Input: part model. Units: mm. Frame: model coordinates. Coordinates: 2 decimals unless noted, no trailing zeros. Write each loop counter-clockwise with the first axis right and the second up, starting at its lowest first coordinate (ties: lowest second). Pieces come first, ordered by that corner, then holes.
1) Draft query along X for faces 1 (the flat face through (-6, 0, -3)), 2 (the cylindrical face through (-5.49, 0.2, -7.62)), 3 (the cylindrical face through (-1.59, 0.2, -3.16)). Return one class per face: pulls with the +X half, pulls with the -X half, needs draft (parallel to the pull), parting line crosses it, or undercut.
2) Section query D-D (x = -4.04). Output: boundary loops of the cut face in (y, z).
3) Section query C-C (y = 0.1). Output: boundary loops of the cut face in (x, z).
4) Line query: L1, parallel to Z at x = -8.25, y = 0.3; L2, parallel to Z at x = -4.04, y = 0.15; L3, parallel to X at y = 0.1, z = -2.75. Output: solid intervals per line, ascending.
5) Section query A-A (x = -11). Output: boundary loops of the cut face in (y, z), then the cut area to 3 significant figures.
6) Section query B-B (z = -3). Output: boundary loops of the cut face in (x, y).
Autodesk Inventor part; units mm, degrees
ref_plane "YZ Plane" through (0, 0, 0) normal (1, 0, 0) x (0, 1, 0)
ref_plane "XZ Plane" through (0, 0, 0) normal (0, 1, 0) x (-1, 0, 0)
ref_plane "XY Plane" through (0, 0, 0) normal (0, 0, 1) x (1, 0, 0)
sketch "Sketch1" plane through (0, 0, 0) normal (0, 1, 0) x (-1, 0, 0)
  line L0 (5, -3.567) -> (5, 0.033)
  line L1 (5, 0.033) -> (0, 0.033)
  line L2 (5.2265, -7.8894) -> (5, -3.567)
  line L3 (5.2265, -0.5894) -> (5, 0.033)
  line L4 (0, -3.567) -> (0, 0.033)
  line L5 (5, -3.567) -> (0, -3.567)
  line L6 (5.2265, -0.1894) -> (12.9265, -0.1894)
  line L7 (12.9265, -0.1894) -> (12.9265, -7.8894)
  line L8 (12.9265, -7.8894) -> (5.2265, -7.8894)
  line L9 (5.2265, -7.8894) -> (5.2265, -0.1894)
  line L10 (5.2265, -0.5894) -> (5.2265, -7.8894) construction
  line L11 (5.2265, -4.2394) -> (11.8919, -4.2394) construction
  line L12 (11.7265, -6.6894) -> (6.4265, -6.6894)
  line L13 (6.4265, -6.6894) -> (6.4265, -1.3894)
  line L14 (6.4265, -1.3894) -> (11.7265, -1.3894)
  line L15 (11.7265, -1.3894) -> (11.7265, -6.6894)
  point P0 (6.1218, -0.1118)
  point P1 (5.2265, -0.5894)
  point P2 (5.4261, -0.5894)
  dimension "d9" = 3.6
  dimension "d10" = 160
  dimension "d12" = 93
  dimension "d18" = 3.65
  dimension "d20" = 1.2
  dimension "d22" = 1.2
  dimension "d28" = 5
  dimension "d39" = 5.3
  dimension "d40" = 5.3
  dimension "d41" = 1.2
  dimension "d42" = 1.2
extrude "Extrusion1" add sketch "Sketch1" along normal blind 0.4
fillet "Fillet3" radius 1 4 edges at (-12.9265, 0.2, -0.1894) (-5.2265, 0.2, -0.1894) (-5.2265, 0.2, -7.8894) (-12.9265, 0.2, -7.8894)
fillet "Fillet4" radius 0.2 4 edges at (-6.4265, 0.2, -6.6894) (-11.7265, 0.2, -6.6894) (-11.7265, 0.2, -1.3894) (-6.4265, 0.2, -1.3894)
fillet "Fillet6" radius 0.2 4 edges at (-5, 0.2, 0.033) (0, 0.2, 0.033) (0, 0.2, -3.567) (-5, 0.2, -3.567)
sketch "Sketch2" plane through (0, 0.4, 0) normal (0, 1, 0) x (1, 0, 0)
  line L0 (0, 0.167) -> (0, 3.367)
  circle A0 centre (-4.04, 2.467) radius 0.7
  circle A1 centre (-1.5, 2.467) radius 0.7
  line L1 (-4.04, 2.467) -> (-1.5, 2.467) construction
  line L2 (-4.86, -0.033) -> (-0.2, -0.033)
  line L3 (-0.2, 3.567) -> (-4.8102, 3.567)
  point P0 (0, 0)
  dimension "d29" = 1.4
  dimension "d31" = 2.54
  dimension "d32" = 1.5
  dimension "d38" = 1.1
extrude "Extrusion2" cut sketch "Sketch2" against normal blind 0.4
fillet "Fillet8" [suppressed]
fillet "Fillet9" radius 2 1 edges at (-5.2265, 0.2, -0.5894)
equation "\"d18\" = 0.5 * d15"
properties part number "PCB_arm"
Answer:
1. face 1: needs draft
1. face 2: pulls with the +X half
1. face 3: undercut
2. outline: (0, -3.57) - (0.4, -3.57) - (0.4, -3.17) - (0, -3.17) - close; (0, -1.77) - (0.4, -1.77) - (0.4, 0.03) - (0, 0.03) - close
3. outline: (-12.93, -6.89) arc R1 ccw to (-11.93, -7.89) - (-6.18, -7.89) arc R1 ccw to (-5.18, -6.94) - (-5.01, -3.76) arc R0.2 cw to (-4.81, -3.57) - (-0.2, -3.57) arc R0.2 ccw to (0, -3.37) - (0, -0.17) arc R0.2 ccw to (-0.2, 0.03) - (-4.86, 0.03) arc R0.2 ccw to (-5.05, -0.1) arc R2 cw to (-5.92, -0.2) arc R1 ccw to (-6.03, -0.19) - (-11.93, -0.19) arc R1 ccw to (-12.93, -1.19) - close; hole (-11.73, -6.49) arc R0.2 ccw to (-11.53, -6.69) - (-6.63, -6.69) arc R0.2 ccw to (-6.43, -6.49) - (-6.43, -1.59) arc R0.2 ccw to (-6.63, -1.39) - (-11.53, -1.39) arc R0.2 ccw to (-11.73, -1.59) - close; hole circle Ø1.4 at (-4.04, -2.47); hole circle Ø1.4 at (-1.5, -2.47)
4. L1: z = -7.89 to -6.69, -1.39 to -0.19
4. L2: z = -3.57 to -3.17, -1.77 to 0.03
4. L3: x = -12.93 to -11.73, -6.43 to -4.68, -3.4 to -2.14, -0.86 to 0
5. outline: (0, -7.89) - (0.4, -7.89) - (0.4, -6.69) - (0, -6.69) - close; (0, -1.39) - (0.4, -1.39) - (0.4, -0.19) - (0, -0.19) - close
5. area: 0.960 mm2
6. outline: (-12.93, 0) - (-11.73, 0) - (-11.73, 0.4) - (-12.93, 0.4) - close; (-6.43, 0) - (-4.49, 0) - (-4.49, 0.4) - (-6.43, 0.4) - close; (-3.59, 0) - (-1.95, 0) - (-1.95, 0.4) - (-3.59, 0.4) - close; (-1.05, 0) - (0, 0) - (0, 0.4) - (-1.05, 0.4) - close
